```python
from build123d import *

# Parameters (mm, degrees)
F0_W     = 60
F0_H     = 110
F1_DEPTH = 50
F3_DEPTH = 60.001
F5_DEPTH = 110.001


with BuildPart() as f1:
    # F0 (on Top) → F1 (new body)
    with BuildSketch(Plane.XY):
        Rectangle(F0_W, F0_H)
    extrude(amount=F1_DEPTH)

    # F2 (on face) → F3 (cut, through all)
    with BuildSketch(Plane.YZ.offset(30)):
        Polygon((-55, 50), (-55, 25), (-13.433757, 25), (1, 50), align=None)
        Polygon((37, 50), (19, 50), (19, 41), (13, 41), (13, 32), (43, 32), (43, 41), (37, 41), align=None)
    extrude(amount=-F3_DEPTH, mode=Mode.SUBTRACT)

    # F4 (on face) → F5 (cut, through all)
    with BuildSketch(Plane.XZ.offset(55)):
        Polygon((25.381198, 8), (30, 0), (30, 8), align=None)
        Polygon((-25.381198, 8), (-30, 8), (-30, 0), align=None)
    extrude(amount=-F5_DEPTH, mode=Mode.SUBTRACT)


solid = f1.part
```
Here's how the part is built. I have some questions about the finished solid (model axes, mm). A direction names the side the tool comes from. Round coordinates to 2 decimals unless told otherwise and drop trailing zeros. Write each loop counter-clockwise with the first axis right and the second up, starting at its lowest first coordinate (ties: lowest second). Pieces come first, ordered by that corner, then holes.
Q1. If we section it at A-A on y = 39: Write out the boundary of the cut face in (x, z), plus the area to 3 significant figures.
Q2. Will these pins go through, and if not, where does the flat tip stop? P1, Ø7, axis at x = -1, z = 37, coming from the -Y side; P2, Ø4.5, axis at x = 8, z = 44.5, coming from the -Y side; P3, Ø10, axis at x = 21.5, z = 37, coming from the -Y side; P4, Ø1.8, axis at x = 2.5, y = 16.5, coming from the -Z side.
Q3. If we section it at B-B on x = -5: Write out the boundary of the cut face in (y, z).
Q4. Which directions (+Z, -Z, +X, -X, +Y, -Y) give clear straight access to the entire face, cutting with the end or side of a thin tool? Please do faces 1 (the flat face through (0, 37, 45)), 2 (the flat face through (-27.723, -0.77, 3.944)), 3 (the flat face through (0, 40, 41)).
Q5. Please list where these lines run through material, in increasing order: probe 1 along Z at (x, y) = (10, 17); probe 2 along Z at (x, y) = (22, 31.5); probe 3 along Y at (x, z) = (10.5, 45.5).
Q6. If we section it at C-C on y = -11.5: Write out the boundary of the cut face in (x, z).
Q7. If we section it at D-D on z = 4.5: Write out the boundary of the cut face in (x, y).
Q8. If we mould it in two halves opening along Z, with no side actions, what happens to faces 4 (the flat face through (30, 11, 24)), 5 (the flat face through (0.42, -6.318, 37.325)), 6 (the flat face through (27.658, -0.77, 4.056))? For each: +Z half, -Z half, draft (parallel to the pull), parting line (faces both ways), or undercut.
Answer below:
1. outline: (-30, 0) - (30, 0) - (25.38, 8) - (30, 8) - (30, 32) - (-30, 32) - (-30, 8) - (-25.38, 8) - close; (-30, 41) - (30, 41) - (30, 50) - (-30, 50) - close
1. area: 2,420 mm2
2. P1: stops at y = -8.53
2. P2: stops at y = -3.47
2. P3: stops at y = -9.39
2. P4: stops at z = 0
3. outline: (-55, 0) - (55, 0) - (55, 50) - (37, 50) - (37, 41) - (43, 41) - (43, 32) - (13, 32) - (13, 41) - (19, 41) - (19, 50) - (1, 50) - (-13.43, 25) - (-55, 25) - close
4. face 1: +Z, +X, -X
4. face 2: -X, +Y, -Y
4. face 3: +X, -X
5. probe 1: z = 0 to 32, 41 to 50
5. probe 2: z = 0 to 32
5. probe 3: y = -1.6 to 19, 37 to 55
6. outline: (-30, 0) - (30, 0) - (25.38, 8) - (30, 8) - (30, 28.35) - (-30, 28.35) - (-30, 8) - (-25.38, 8) - close
7. outline: (-27.4, -55) - (27.4, -55) - (27.4, 55) - (-27.4, 55) - close
8. face 4: draft
8. face 5: +Z half
8. face 6: undercut
